Source: CAD feature listing. Evaluate the final solid. Frame: model axes, mm. A direction names the side the tool comes from. Give positions to 0.01 mm unless a question says otherwise; leave off trailing zeros. Loops run counter-clockwise (first coordinate to the right, second up) from the corner with the lowest first, then second, coordinate; pieces in that order, holes last.
Autodesk Inventor part; units mm, degrees
ref_plane "YZ Plane" through (0, 0, 0) normal (1, 0, 0) x (0, 1, 0)
ref_plane "XZ Plane" through (0, 0, 0) normal (0, 1, 0) x (-1, 0, 0)
ref_plane "XY Plane" through (0, 0, 0) normal (0, 0, 1) x (1, 0, 0)
sketch "Sketch1" plane through (0, 0, 0) normal (0, 0, 1) x (1, 0, 0)
  line L0 (0, 0) -> (19, 0)
  line L1 (19, 0) -> (19, 100)
  line L2 (19, 100) -> (0, 100)
  line L3 (0, 100) -> (0, 0)
  dimension "d0" = 19
  dimension "d1" = 100
extrude "Extrusion1" add sketch "Sketch1" along normal blind 19
sketch "Sketch3" plane through (0, 100, 0) normal (0, 1, 0) x (1, 0, 0)
  line L0 (19, 0) -> (0, 0)
  line L1 (0, 0) -> (0, -19)
  line L2 (19, -19) -> (0, -19)
  line L3 (19, 0) -> (19, -19)
  line L4 (1.5, -17.5) -> (1.5, -1.5)
  line L5 (1.5, -1.5) -> (17.5, -1.5)
  line L6 (17.5, -1.5) -> (17.5, -17.5)
  line L7 (17.5, -17.5) -> (1.5, -17.5)
  point P0 (0, 0)
  dimension "d4" = 1.5
extrude "Extrusion2" cut sketch "Sketch3" against normal through all contours L4 L5 L6 L7
properties part number "C006" material "Aluminum 6061"
(1) Reachability of faces 1 (the flat face through (9, 51, 0)), 2 (the flat face through (17.5, 51, 9)) from +Z, -Z, +X, -X, +Y, -Y: full face, straight path, thin tool, end or side. Return the list, or none.
A:
face 1: -Z, +X, -X, +Y, -Y
face 2: +Y, -Y
(2) Section C-C, the plane y = 23.5. Return the cut outline in (x, z), then the cut area to 3 significant figures.
A:
outline: (0, 0) - (19, 0) - (19, 19) - (0, 19) - close; hole (1.5, 1.5) - (17.5, 1.5) - (17.5, 17.5) - (1.5, 17.5) - close
area: 105 mm2
(3) First-contact query: pin 1 (4 mm diameter, centred on x = 8.5, y = 87.5, fed in from -Z). Flat tip, straight axial feed; report the tip coordinate or a pass-through.
A:
pin 1: stops at z = 0
(4) Ray query, line 1 along Z through (x, y) = (13.25, 61). Return the intervals inside material, ascending.
A:
line 1: z = 0 to 1.5, 17.5 to 19
(5) Section B-B, the plane x = 5.75. Return the cut outline in (y, z).
A:
outline: (0, 0) - (100, 0) - (100, 1.5) - (0, 1.5) - close; (0, 17.5) - (100, 17.5) - (100, 19) - (0, 19) - close
(6) Section A-A, the plane z = 11. Return the cut outline in (x, y), then the cut area to 3 significant figures.
A:
outline: (0, 0) - (1.5, 0) - (1.5, 100) - (0, 100) - close; (17.5, 0) - (19, 0) - (19, 100) - (17.5, 100) - close
area: 300 mm2
(7) Mould query, pull axis X, two halves, no side actions, for faces 3 (the flat face through (0, 51, 9)), 4 (the flat face through (18, 100, 9)), 5 (the flat face through (1.5, 51, 10)). Classes: pulls with the +X half, pulls with the -X half, needs draft (parallel to the pull), parting line crosses it, or undercut.
A:
face 3: pulls with the -X half
face 4: needs draft
face 5: undercut
